```python
from build123d import *

# Parameters (mm, degrees)
F2_R      = 25
F3_DEPTH  = 41.5
F4_R      = 12.5
F5_DEPTH  = 30
F6_R      = 2.5
F7_DEPTH  = 62.501
F8_R      = 4.5
F9_DEPTH  = 13.5010001
F12_DEPTH = 14


with BuildPart() as f1:
    # F0 (on Front) → F1 (revolve)
    with BuildSketch(Plane.XZ):
        Polygon((10.5, 62.5), (0, 62.5), (0, 35), (-3, 35), (-3, 16), (247, 16), (247, 25), (10.5, 25), align=None)
    revolve(axis=Axis((-11.2489545718, 0, 0), (-1, 0, 0)))

    # F2 (on face) → F3 (join)
    with BuildSketch(Plane.YZ.offset(10.5)):
        with BuildLine():
            Line((26, -13.9373598648), (26, 37.3396572025))
            ThreePointArc((26, 37.3396572025), (0, 45.5), (-26, 37.3396572025))
            Line((-26, 37.3396572025), (-26, -13.9373598648))
            ThreePointArc((-26, -13.9373598648), (0, -29.5), (26, -13.9373598648))
        make_face()
        Circle(F2_R, mode=Mode.SUBTRACT)
    extrude(amount=F3_DEPTH)

    # F4 (on Front) → F5 (cut, symmetric)
    with BuildSketch(Plane.XZ):
        with Locations((30, 22.2058613113)):
            Circle(F4_R)
    extrude(amount=F5_DEPTH, both=True, mode=Mode.SUBTRACT)

    # F6 (on Front) → F7 (cut, through all)
    with BuildSketch(Plane.XZ):
        with Locations((237, 0)):
            Circle(F6_R)
    extrude(amount=-F7_DEPTH, mode=Mode.SUBTRACT)

    # F8 (on face) → F9 (cut, through all)
    with BuildSketch(Plane.YZ.offset(10.5)):
        with Locations((-28, 48.4974226119)):
            Circle(F8_R)
        with Locations((56, 0)):
            Circle(F8_R)
        with Locations((-28, -48.4974226119)):
            Circle(F8_R)
    extrude(amount=-F9_DEPTH, mode=Mode.SUBTRACT)

    # F11 (on offset) → F12 (join)
    with BuildSketch(Plane(origin=(24, 0, 0), x_dir=(0, -1, 0), z_dir=(-1, 0, 0))):
        with BuildLine():
            Line((-13, 2.5), (-15.8034806293, 2.5))
            ThreePointArc((-15.8034806293, 2.5), (-16, 0), (-15.8034806293, -2.5))
            Line((-15.8034806293, -2.5), (-13, -2.5))
            Line((-13, -2.5), (-13, 2.5))
        make_face()
        with BuildLine():
            ThreePointArc((15.8034806293, -2.5), (16, 0), (15.8034806293, 2.5))
            Line((15.8034806293, 2.5), (13, 2.5))
            Line((13, 2.5), (13, -2.5))
            Line((13, -2.5), (15.8034806293, -2.5))
        make_face()
    extrude(amount=-F12_DEPTH)


solid = f1.part
```
Verification items for the finished model (mm, model axes). A direction names the side the tool comes from. Give positions to 0.01 mm unless a question says otherwise; leave off trailing zeros. Order: outer loops, then holes, each group sorted by start corner. A loop starts at its lowest first (then second) coordinate and runs counter-clockwise, first axis right, second up. Notation, with made-up numbers: (4, 10) -> (12, 10) arc R14 ccw to (12, 17) -> close; hole circle Ø7 at (29, 81.5). An arc over 180 degrees is marked (long way). One line per item, written item: value.
(1) Scan lines: line 1 along Z through (x, y) = (8, -28); line 2 along Z through (x, y) = (30, 0.5); line 3 along X through (y, z) = (1.5, -38.5). Record each from-to range of solid material in increasing order. Write a range as [from, to].
Final values:
line 1: [-55.88, -53], [-44, 44], [53, 55.88]
line 2: [-29.5, -15.99], [34.71, 45.5]
line 3: [0, 10.5]
(2) Sectioned sample at A-A on y = 22. Record the cut outline in (x, z).
Final values:
outline: (-3, -27.22) -> (0, -27.22) -> (0, -58.5) -> (10.5, -58.5) -> (10.5, -19.65) -> (52, -19.65) -> (52, -11.87) -> (247, -11.87) -> (247, 11.87) -> (52, 11.87) -> (52, 39.83) -> (10.5, 39.83) -> (10.5, 58.5) -> (0, 58.5) -> (0, 27.22) -> (-3, 27.22) -> close; hole circle Ø25 at (30, 22.21); hole circle Ø5 at (237, 0)
(3) Sectioned sample at C-C on z = 0. Count the separate pieces of the cut face and the enclosed holes in it, then the cut area to 4 significant figures.
Final values:
separate pieces: 4
enclosed holes: 0
area: 5,375 mm^2
(4) Gauge pin test, flat ends, axial feed: pin 1 (5.5 mm diameter, centred on x = 28, z = 0.5, fed in from +Y); pin 2 (2.5 mm diameter, centred on y = -14.5, z = -1, fed in from +X); pin 3 (2 mm diameter, centred on x = 129.5, z = -18.5, fed in from -Y). Record the tip position at first contact, or that the pin passes through.
Final values:
pin 1: y = 26
pin 2: x = 38
pin 3: y = -17.85
(5) Sectioned sample at D-D on y = 56. Record the cut outline in (x, z), then the cut area to 3 significant figures.
Final values:
outline: (0, -27.75) -> (10.5, -27.75) -> (10.5, -4.5) -> (0, -4.5) -> close; (0, 4.5) -> (10.5, 4.5) -> (10.5, 27.75) -> (0, 27.75) -> close
area: 488 mm^2
(6) Draft check along Y on faces 5 (the face through (0, -27, 27)), 6 (the face through (5.18, 2.75, -62.44)), 7 (the face through (5.324, 60.292, 1.352)). Enter one of: pulls with the +Y half, pulls with the -Y half, needs draft (parallel to the pull), parting line crosses it, or undercut.
Final values:
face 5: needs draft
face 6: parting line crosses it
face 7: undercut
(7) Tool access check on faces 1 (the face through (239.385, 20.339, 0.751)), 2 (the face through (31, -26, 6)), 3 (the face through (30.96, -0.445, -29.497)), 4 (the face through (31, 13, 0)). Record the directions out of +Z, -Z, +X, -X, +Y, -Y that give a thin tool (end or side, any length) a straight path to the whole face; none if there is none.
Final values:
face 1: +Y
face 2: +Z, -Z, +X, -Y
face 3: -Z, +X
face 4: +X, -X
(8) Sectioned sample at B-B on x = 194. Record the cut outline in (y, z).
Final values:
outline: circle Ø50 at (0, 0); hole circle Ø32 at (0, 0)
